Input: part model. Units: mm. Frame: model coordinates. A direction names the side the tool comes from. Coordinates: 2 decimals unless noted, no trailing zeros. Order: outer loops, then holes, each group sorted by start corner. A loop starts at its lowest first (then second) coordinate and runs counter-clockwise, first axis right, second up. Notation, with made-up numbers: (-5, 19.5) -> (16, 19.5) arc R24 cw to (16, 48.5) -> close; hole circle Ø5 at (-27, 15). An arc over 180 degrees is marked (long way). One line per question, with ' | ' between items.
```python
from build123d import *

# Parameters (mm, degrees)
BOX001_W              = 1.1
BOX001_H              = 1
BOX001_DEPTH          = 1
ARRAY_X_COUNT         = 4
ARRAY_X_PITCH         = 2
BOX_W                 = 8
BOX_H                 = 8
BOX_DEPTH             = 1
CLONE_PLACEMENT_ANGLE = 180


with BuildPart() as array:
    # Box001 → Box001 (new body)
    with BuildSketch(Plane(origin=(17.86, 30.4267, 0), x_dir=(1, 0, 0), z_dir=(0, 0, 1))):
        with Locations((0.55, 0.5)):
            Rectangle(BOX001_W, BOX001_H)
    extrude(amount=BOX001_DEPTH)

    # Array X: Array ×4


with BuildPart() as array_1:
    add(array.part)
    with Locations(*[(i * ARRAY_X_PITCH, 0, 0) for i in range(1, ARRAY_X_COUNT)]):
        add(array.part)


with BuildPart() as array_2:
    # Array placement: moved
    add(array_1.part.moved(Location((-0.05, 0, 0))))


with BuildPart() as fingersrev:
    # Box → Box (new body)
    with BuildSketch(Plane(origin=(17.86, 30.4267, 0), x_dir=(1, 0, 0), z_dir=(0, 0, 1))):
        with Locations((4, 4)):
            Rectangle(BOX_W, BOX_H)
    extrude(amount=BOX_DEPTH)

    # Cut: cut Array
    add(array_2.part, mode=Mode.SUBTRACT)


with BuildPart() as fingersrev_1:
    # Clone placement: moved
    add(fingersrev.part.moved(Location((43.72, 55.8434, 0))).rotate(Axis((43.72, 55.8434, 0), (0, 0, 1)), CLONE_PLACEMENT_ANGLE))


solid = fingersrev_1.part
```
1. Pin query (flat end, axial travel): pin 1 Ø0.5 at (y, z) = (25, 0.5) entering from +X. Return the tip coordinate at first contact, or that it passes through.
Recorded:
pin 1: stops at x = 24.81
2. Access query for faces 5 (the face through (21.91, 24.9, 0.5)), 6 (the face through (24.81, 24.9, 0.5)), 7 (the face through (22.4, 25.417, 0.5)). Directions: +Z, -Z, +X, -X, +Y, -Y. A direction counts if a zero-diameter tool reaches every point of the face in a straight line with its end or side. Return the directions, or none.
Recorded:
face 5: +Z, -Z, +Y | face 6: +Z, -Z, +X, +Y | face 7: +Z, -Z, +X, -X, +Y
3. Cut plane C-C, the plane x = 23.25. Return loops of the section in (y, z), and give its area (3 significant figures).
Recorded:
outline: (17.42, 0) -> (24.42, 0) -> (24.42, 1) -> (17.42, 1) -> close | area: 7.00 mm^2
4. Cut plane B-B, the plane z = 0.8. Return loops of the section in (x, y), and give its area (4 significant figures).
Recorded:
outline: (17.86, 17.42) -> (25.86, 17.42) -> (25.86, 24.42) -> (24.81, 24.42) -> (24.81, 25.42) -> (23.91, 25.42) -> (23.91, 24.42) -> (22.81, 24.42) -> (22.81, 25.42) -> (21.91, 25.42) -> (21.91, 24.42) -> (20.81, 24.42) -> (20.81, 25.42) -> (19.91, 25.42) -> (19.91, 24.42) -> (18.81, 24.42) -> (18.81, 25.42) -> (17.86, 25.42) -> close | area: 59.65 mm^2
5. Cut plane A-A, the plane y = 25. Return loops of the section in (x, z).
Recorded:
outline: (17.86, 0) -> (18.81, 0) -> (18.81, 1) -> (17.86, 1) -> close; (19.91, 0) -> (20.81, 0) -> (20.81, 1) -> (19.91, 1) -> close; (21.91, 0) -> (22.81, 0) -> (22.81, 1) -> (21.91, 1) -> close; (23.91, 0) -> (24.81, 0) -> (24.81, 1) -> (23.91, 1) -> close
6. Ray query, line 1 (X direction, y = 24.75, z = 0.1); line 2 (Y direction, x = 19, z = 0.85). Return the intervals inside material, ascending. Write a range as [from, to].
Recorded:
line 1: x = [17.86, 18.81], [19.91, 20.81], [21.91, 22.81], [23.91, 24.81] | line 2: y = [17.42, 24.42]
7. Mould query, pull axis X, two halves, no side actions, for faces 1 (the face through (22.81, 24.9, 0.5)), 2 (the face through (23.91, 24.9, 0.5)), 3 (the face through (25.86, 21, 0.5)), 4 (the face through (21.9, 17.417, 0.5)). Classes: released by +X, released by -X, zero draft, split by the parting line, or undercut.
Recorded:
face 1: undercut | face 2: undercut | face 3: released by +X | face 4: zero draft
